from build123d import *

# Parameters (mm, degrees)
BOSS_EXTRUDE1_DEPTH = 8.5
FILLET1_R           = 3
SKETCH2_W           = 8
SKETCH2_H           = 3
BOSS_EXTRUDE2_DEPTH = 17
SKETCH3_R           = 2.25
CUT_EXTRUDE1_DEPTH  = 4


with BuildPart() as part:
    # Sketch1 → Boss-Extrude1 (new body, symmetric)
    with BuildSketch(Plane(origin=(0, 0, 0), x_dir=(1, 0, 0), z_dir=(0, 1, 0))):
        Polygon((0, 0), (0, 10), (8, 11.410615846), (6.089870046, 22.243501129), (30, 45.904610688), (24.86969785, 60), (40, 60), (40, 0), align=None)
        Polygon((16, 8), (32, 8), (32, 36.628833574), (16, 20.795471159), align=None, mode=Mode.SUBTRACT)
    extrude(amount=BOSS_EXTRUDE1_DEPTH, both=True)

    # Fillet1
    fillet1_edges = [part.edges().sort_by_distance(p)[0] for p in [
        (0, 0, -10),
        (6.089870046, 0, -22.243501129),
        (24.86969785, 0, -60),
        (40, 0, -60),
        (16, 0, -20.795471159),
        (16, 0, -8),
        (32, 0, -8),
        (32, 0, -36.628833574),
    ]]
    fillet(fillet1_edges, radius=FILLET1_R)

    # Sketch2 → Boss-Extrude2 (add)
    with BuildSketch(Plane(origin=(0, 8.5, 0), x_dir=(1, 0, 0), z_dir=(0, 1, 0))):
        with Locations((-4, 1.5)):
            Rectangle(SKETCH2_W, SKETCH2_H)
        with Locations((44, 1.5)):
            Rectangle(SKETCH2_W, SKETCH2_H)
    extrude(amount=-BOSS_EXTRUDE2_DEPTH)

    # Sketch3 → Cut-Extrude1 (cut, through all)
    with BuildSketch(Plane(origin=(0, 0, -3), x_dir=(-1, 0, 0), z_dir=(0, 0, -1))):
        with Locations((4, -4.5)):
            Circle(SKETCH3_R)
        with Locations((4, 4.5)):
            Circle(SKETCH3_R)
        with Locations((-44, 4.5)):
            Circle(SKETCH3_R)
        with Locations((-44, -4.5)):
            Circle(SKETCH3_R)
    extrude(amount=-CUT_EXTRUDE1_DEPTH, mode=Mode.SUBTRACT)


solid = part.part
Here's how the part is built. I have some questions about the finished solid (model axes, mm). A direction names the side the tool comes from. Round coordinates to 2 decimals unless told otherwise and drop trailing zeros. Write each loop counter-clockwise with the first axis right and the second up, starting at its lowest first coordinate (ties: lowest second). Pieces come first, ordered by that corner, then holes.
1. Suppose I cut it at A-A (x = 44). List the corners of the cut face in (y, z) for me.
2. For faces 1 (the flat face through (32, 0, -20)), 2 (the flat face through (5.201, 0.119, -10.917)), 3 (the flat face through (40, 0, -30)), 4 (the flat face through (-4, 0, -3)), which set-ups out of +Z, -Z, +X, -X, +Y, -Y let a thin tool reach every point of the face, with its end or its side?
3. If we mould it in two halves opening along X, with no side actions, what happens to faces 5 (the cylindrical face through (30.2, 0.12, -32.19)), 6 (the flat face through (0, 0, -5)), 7 (the flat face through (48, 0, -1))? For each: released by +X, released by -X, zero draft, split by the parting line, or undercut.
4. I need wall thicknesses on L1, parallel to Y at x = 44, z = -0.8; L2, parallel to X at y = 3, z = -11.5; L3, parallel to X at y = -6.5, z = -2.5. Which ranges of each line are inside material? Lowest first, please.
5. Suppose I cut it at C-C (y = 4.5). State how many separate pieces and enclosed holes the cut face has, and give its area (3 significant figures).
6. Suppose I cut it at B-B (y = 7.75). List the corners of the cut face in (x, z) for me, and give its area (3 significant figures).
7. Will these pins go through, and if not, where does the flat tip stop? pin 1 Ø10 at (y, z) = (-3.5, -26) entering from -X; pin 2 Ø10 at (y, z) = (5, -47.5) entering from +X; pin 3 Ø4 at (x, y) = (-2.5, -0.5) entering from -Z.
Answer sheet:
1. outline: (-8.5, -3) - (-6.75, -3) - (-6.75, 0) - (-8.5, 0) - close; (-2.25, -3) - (2.25, -3) - (2.25, 0) - (-2.25, 0) - close; (6.75, -3) - (8.5, -3) - (8.5, 0) - (6.75, 0) - close
2. face 1: +Y, -Y
2. face 2: -X, +Y, -Y
2. face 3: -Z, +X, +Y, -Y
2. face 4: -Z, -X, +Y, -Y
3. face 5: undercut
3. face 6: released by -X
3. face 7: released by +X
4. L1: y = -8.5 to -6.75, -2.25 to 2.25, 6.75 to 8.5
4. L2: x = 7.98 to 16, 32 to 40
4. L3: x = -8 to -5.03, -2.97 to 42.97, 45.03 to 48
5. separate pieces: 3
5. enclosed holes: 1
5. area: 1,200 mm2
6. outline: (-8, -3) - (0, -3) - (0, -7.48) arc R3 ccw to (2.48, -10.44) - (8, -11.41) - (6.36, -20.7) arc R3 ccw to (7.21, -23.35) - (30, -45.9) - (26.34, -55.97) arc R3 ccw to (29.15, -60) - (37, -60) arc R3 ccw to (40, -57) - (40, -3) - (48, -3) - (48, 0) - (-8, 0) - close; hole (16, -19.54) arc R3 ccw to (16.89, -21.68) - (26.89, -31.57) arc R3 ccw to (32, -29.44) - (32, -11) arc R3 ccw to (29, -8) - (19, -8) arc R3 ccw to (16, -11) - close
6. area: 1,230 mm2
7. pin 1: stops at x = 6.32
7. pin 2: stops at x = 40
7. pin 3: stops at z = -3
